Can you work these out from the model? Positions are in its coordinate system, mm. A direction names the side the tool comes from. Give positions to 0.01 mm unless a question says otherwise; leave off trailing zeros. Order: outer loops, then holes, each group sorted by start corner. A loop starts at its lowest first (then second) coordinate and runs counter-clockwise, first axis right, second up. Notation, with made-up numbers: (39.5, 33.5) -> (43.5, 33.5) arc R18 ccw to (43.5, 47.5) -> close; hole circle Ø11 at (-12, 77). An arc over 180 degrees is marked (long way). Answer as CSV lines item,"result".
```python
from build123d import *

# Parameters (mm, degrees)
SKETCH1_W           = 1350
SKETCH1_H           = 300
EXTRUDE1_DEPTH      = 30
SKETCH2_R           = 12
CUT_EXTRUDE1_DEPTH  = 31
EXTRUDE2_DEPTH      = 15
LPATTERN1_COUNT     = 2
LPATTERN1_PITCH     = 130
LPATTERN1_COL_COUNT = 2
LPATTERN1_COL_PITCH = 130


with BuildPart() as part:
    # Sketch1 → Extrude1 (new body)
    with BuildSketch(Plane.XY):
        with Locations((50.339261683, -50.554392858)):
            Rectangle(SKETCH1_W, SKETCH1_H)
    extrude(amount=EXTRUDE1_DEPTH)

    # Sketch2 → Cut-Extrude1 (cut, through all)
    with BuildSketch(Plane.XY.offset(30)):
        with Locations((675.339261683, 24.445607142)):
            Circle(SKETCH2_R)
        with Locations((675.339261683, -125.554392858)):
            Circle(SKETCH2_R)
        with Locations(Location((-574.660738317, -125.554392858, 0), (0, 0, 180))):  # turned: the seam where the file's is
            Circle(SKETCH2_R)
        with Locations(Location((-574.660738317, 24.445607142, 0), (0, 0, 180))):  # turned: the seam where the file's is
            Circle(SKETCH2_R)
    extrude(amount=-CUT_EXTRUDE1_DEPTH, mode=Mode.SUBTRACT)

    # Sketch3 → Extrude2 (add, symmetric)
    with BuildSketch(Plane(origin=(-624.660738317, -50.554392858, 0), x_dir=(1, 0, 0), z_dir=(0, -1, 0))):
        Polygon((52.834900275, 30), (52.834900275, 127.16727695), (370.2, 351.189991199), (979.8, 351.189991199), (1297.165099725, 127.16727695), (1297.165099725, 30), align=None)
    extrude2 = extrude(amount=EXTRUDE2_DEPTH, both=True)

    # LPattern1: Extrude2 ×2
    with Locations(*[(0, -i * LPATTERN1_PITCH, 0) for i in range(1, LPATTERN1_COUNT)]):
        add(extrude2)

    # LPattern1 col: Extrude2 ×2
    with Locations(*[(0, i * LPATTERN1_COL_PITCH, 0) for i in range(1, LPATTERN1_COL_COUNT)]):
        add(extrude2)


solid = part.part
```
Item 1: Imagine slicing it at A-A, the plane z = 272. Please give me the cut outline in (x, y).
Numbers:
outline,"(-366.65, -195.55) -> (467.32, -195.55) -> (467.32, -165.55) -> (-366.65, -165.55) -> close; (-366.65, -65.55) -> (467.32, -65.55) -> (467.32, -35.55) -> (-366.65, -35.55) -> close; (-366.65, 64.45) -> (467.32, 64.45) -> (467.32, 94.45) -> (-366.65, 94.45) -> close"
Item 2: For faces 1 (the flat face through (672.504, -51, 79)), 2 (the flat face through (59, 64.446, 157)), 3 (the flat face through (59, 94.446, 157)), which set-ups out of +Z, -Z, +X, -X, +Y, -Y let a thin tool reach every point of the face, with its end or its side?
Numbers:
face 1,"+Z, +X, +Y, -Y"
face 2,"+Z, +X, -X"
face 3,"+Z, +X, -X, +Y"
Item 3: Imagine slicing it at D-D, the plane z = 205.5. Please give me the cut outline in (x, y), then the cut area to 3 significant figures.
Numbers:
outline,"(-460.85, -195.55) -> (561.53, -195.55) -> (561.53, -165.55) -> (-460.85, -165.55) -> close; (-460.85, -65.55) -> (561.53, -65.55) -> (561.53, -35.55) -> (-460.85, -35.55) -> close; (-460.85, 64.45) -> (561.53, 64.45) -> (561.53, 94.45) -> (-460.85, 94.45) -> close"
area,"92,000 mm²"
Item 4: For pin 1 (24 mm diameter, centred on y = -55.5, z = 79.5, fed in from +X); pin 2 (21.5 mm diameter, centred on x = -574.66, y = 24.45, fed in from -Z); pin 3 (6 mm diameter, centred on x = 208.5, z = 57, fed in from -Y); pin 4 (10 mm diameter, centred on x = 263, y = -117, fed in from +Z), each with a flat end and sliding along its axis, tell me the tip position at first contact or that it passes through.
Numbers:
pin 1,"stops at x = 672.5"
pin 2,"passes through"
pin 3,"stops at y = -195.55"
pin 4,"stops at z = 30"
Item 5: We'd pull the mould along X, two halves only. Please class faces 4 (the flat face through (46, 79, 351.19)), 5 (the cylindrical face through (-562.672, 23.918, 15.21)), 6 (the flat face through (-624.661, -53, 15)): released by +X, released by -X, zero draft, split by the parting line, or undercut.
Numbers:
face 4,"zero draft"
face 5,"undercut"
face 6,"released by -X"
Item 6: Imagine slicing it at B-B, the plane x = 44. Please give me the cut outline in (y, z), then the cut area to 3 significant figures.
Numbers:
outline,"(-200.55, 0) -> (99.45, 0) -> (99.45, 30) -> (94.45, 30) -> (94.45, 351.19) -> (64.45, 351.19) -> (64.45, 30) -> (-35.55, 30) -> (-35.55, 351.19) -> (-65.55, 351.19) -> (-65.55, 30) -> (-165.55, 30) -> (-165.55, 351.19) -> (-195.55, 351.19) -> (-195.55, 30) -> (-200.55, 30) -> close"
area,"37,900 mm²"
Item 7: Imagine slicing it at C-C, the plane y = -21. Please give me the cut outline in (x, z).
Numbers:
outline,"(-624.66, 0) -> (725.34, 0) -> (725.34, 30) -> (-624.66, 30) -> close"
Item 8: Please list where these lines run through material, in increasing order: line 1 along Y through (x, z) = (-364, 231.5); line 2 along X through (y, z) = (17.5, 24); line 3 along X through (y, z) = (-54.5, 39).
Numbers:
line 1,"y = -195.55 to -165.55, -65.55 to -35.55, 64.45 to 94.45"
line 2,"x = -624.66 to -584.45, -564.88 to 665.55, 685.12 to 725.34"
line 3,"x = -571.83 to 672.5"
